Build history of the part. All positions in model axes, mm. A direction names the side the tool comes from. Round coordinates to 2 decimals unless told otherwise and drop trailing zeros. Loops run counter-clockwise (first coordinate to the right, second up) from the corner with the lowest first, then second, coordinate; pieces in that order, holes last. Notation, with made-up numbers: (-34.5, 50) -> (-1.5, 50) arc R20 cw to (-1.5, 80) -> close; hole circle Ø9 at (-22.5, 9). An arc over 180 degrees is marked (long way). Put each result on its own line as item: value. Start each with the question number.
Item 1: Cut at C-C, the plane y = 5. List the corners of the cut face in (x, z), plus the area to 3 significant figures.
Item 2: Flat gauge pins, fed straight in: pin 1 Ø5 at (y, z) = (15, -8.5) entering from -X; pin 2 Ø8.5 at (y, z) = (13.5, 8) entering from +X; pin 3 Ø1.9 at (x, z) = (41.5, -40.5) entering from +Y; pin 4 Ø5 at (x, z) = (25, 30.5) entering from -Y. Where does each tip first touch, or does it go through?
Item 3: Tool access for faces 5 (the flat face through (-1, 19, 38)), 6 (the flat face through (-36, 6, 32)), 7 (the flat face through (-39, 19, 1)): list every direction of +Z, -Z, +X, -X, +Y, -Y with a clear straight run to the whole face (end or side of a thin tool).
Item 4: Drill centre lines: probe 1 along Z at (x, y) = (25, 18.7); probe 2 along X at (y, z) = (17.7, 30.5); probe 3 along X at (y, z) = (0.95, -40.5). Where is each one in solid material? Low to high. Write a range as [from, to].
Item 5: Cut at B-B, the plane z = 30.5. List the corners of the cut face in (x, y).
Item 6: Cut at D-D, the plane x = 25. List the corners of the cut face in (y, z), plus the area to 3 significant figures.
Item 7: Cut at A-A, the plane x = 41.5. List the corners of the cut face in (y, z).
Item 8: Pull direction Z, two halves, no side cores. Call faces 1 (the cylindrical face through (-40.76, 1.52, -39.08)), 2 (the flat face through (39, 0, -38)), 3 (the flat face through (39, 1, -44)), 4 (the flat face through (-39, 1, 44)): +Z half, -Z half, draft (parallel to the pull), parting line (faces both ways), or undercut.
```python
from build123d import *

# Parameters (mm, degrees)
SKETCH1_W             = 12
SKETCH1_H             = 12
BOSS_EXTRUDE1_DEPTH   = 3
BOSS_EXTRUDE1_2_DEPTH = 3
BOSS_EXTRUDE1_3_DEPTH = 3
BOSS_EXTRUDE1_4_DEPTH = 3
SKETCH2_W             = 6
SKETCH2_H             = 6
BOSS_EXTRUDE3_DEPTH   = 14
SKETCH3_W             = 78
SKETCH3_H             = 76
BOSS_EXTRUDE4_DEPTH   = 3
CUT_EXTRUDE1_REACH    = 5
SKETCH4_R             = 1.6
CUT_EXTRUDE2_REACH    = 22
SKETCH5_R             = 2.1


with BuildPart() as part:
    # Sketch1 → Boss-Extrude1 (new body)
    with BuildSketch(Plane(origin=(0, 0, 0), x_dir=(1, 0, 0), z_dir=(0, 1, 0))):
        with Locations((-39, -38)):
            Rectangle(SKETCH1_W, SKETCH1_H)
    extrude(amount=BOSS_EXTRUDE1_DEPTH)



with BuildPart() as body_2:
    # Sketch1 → Boss-Extrude1 2 (new body)
    with BuildSketch(Plane(origin=(0, 0, 0), x_dir=(1, 0, 0), z_dir=(0, 1, 0))):
        with Locations((-39, 38)):
            Rectangle(SKETCH1_W, SKETCH1_H)
    extrude(amount=BOSS_EXTRUDE1_2_DEPTH)


with BuildPart() as body_3:
    # Sketch1 → Boss-Extrude1 3 (new body)
    with BuildSketch(Plane(origin=(0, 0, 0), x_dir=(1, 0, 0), z_dir=(0, 1, 0))):
        with Locations((39, 38)):
            Rectangle(SKETCH1_W, SKETCH1_H)
    extrude(amount=BOSS_EXTRUDE1_3_DEPTH)


with BuildPart() as body_4:
    # Sketch1 → Boss-Extrude1 4 (new body)
    with BuildSketch(Plane(origin=(0, 0, 0), x_dir=(1, 0, 0), z_dir=(0, 1, 0))):
        with Locations((39, -38)):
            Rectangle(SKETCH1_W, SKETCH1_H)
    extrude(amount=BOSS_EXTRUDE1_4_DEPTH)


with BuildPart() as part_1:
    add(part.part)

    add(body_2.part)  # Boss-Extrude3 merges body 2

    add(body_3.part)  # Boss-Extrude3 merges body 3

    add(body_4.part)  # Boss-Extrude3 merges body 4
    # Sketch2 → Boss-Extrude3 (add)
    with BuildSketch(Plane(origin=(0, 3, 0), x_dir=(1, 0, 0), z_dir=(0, 1, 0))):
        with Locations((-36, 35)):
            Rectangle(SKETCH2_W, SKETCH2_H)
        with Locations((-36, -35)):
            Rectangle(SKETCH2_W, SKETCH2_H)
        with Locations((36, 35)):
            Rectangle(SKETCH2_W, SKETCH2_H)
        with Locations((36, -35)):
            Rectangle(SKETCH2_W, SKETCH2_H)
    extrude(amount=BOSS_EXTRUDE3_DEPTH)

    # Sketch3 → Boss-Extrude4 (add)
    with BuildSketch(Plane(origin=(0, 17, 0), x_dir=(1, 0, 0), z_dir=(0, 1, 0))):
        Rectangle(SKETCH3_W, SKETCH3_H)
    extrude(amount=BOSS_EXTRUDE4_DEPTH)

    # Sketch4 → Cut-Extrude1 (cut, up to next)
    with BuildSketch(Plane(origin=(0, 3, 0), x_dir=(1, 0, 0), z_dir=(0, 1, 0)), mode=Mode.PRIVATE) as cut_extrude1_sk1:
        with Locations((41.5, -40.5)):
            Circle(SKETCH4_R)
    cut_extrude1_tool1 = extrude(cut_extrude1_sk1.sketch, amount=-CUT_EXTRUDE1_REACH, mode=Mode.PRIVATE) & part_1.part
    add(cut_extrude1_tool1.solids().sort_by_distance((41.5, 3, 40.5))[0], mode=Mode.SUBTRACT)
    # Sketch4 → Cut-Extrude1 (cut, up to next)
    with BuildSketch(Plane(origin=(0, 3, 0), x_dir=(1, 0, 0), z_dir=(0, 1, 0)), mode=Mode.PRIVATE) as cut_extrude1_sk2:
        with Locations((-41.5, 40.5)):
            Circle(SKETCH4_R)
    cut_extrude1_tool2 = extrude(cut_extrude1_sk2.sketch, amount=-CUT_EXTRUDE1_REACH, mode=Mode.PRIVATE) & part_1.part
    add(cut_extrude1_tool2.solids().sort_by_distance((-41.5, 3, -40.5))[0], mode=Mode.SUBTRACT)
    # Sketch4 → Cut-Extrude1 (cut, up to next)
    with BuildSketch(Plane(origin=(0, 3, 0), x_dir=(1, 0, 0), z_dir=(0, 1, 0)), mode=Mode.PRIVATE) as cut_extrude1_sk3:
        with Locations((-41.5, -40.5)):
            Circle(SKETCH4_R)
    cut_extrude1_tool3 = extrude(cut_extrude1_sk3.sketch, amount=-CUT_EXTRUDE1_REACH, mode=Mode.PRIVATE) & part_1.part
    add(cut_extrude1_tool3.solids().sort_by_distance((-41.5, 3, 40.5))[0], mode=Mode.SUBTRACT)
    # Sketch4 → Cut-Extrude1 (cut, up to next)
    with BuildSketch(Plane(origin=(0, 3, 0), x_dir=(1, 0, 0), z_dir=(0, 1, 0)), mode=Mode.PRIVATE) as cut_extrude1_sk4:
        with Locations((41.5, 40.5)):
            Circle(SKETCH4_R)
    cut_extrude1_tool4 = extrude(cut_extrude1_sk4.sketch, amount=-CUT_EXTRUDE1_REACH, mode=Mode.PRIVATE) & part_1.part
    add(cut_extrude1_tool4.solids().sort_by_distance((41.5, 3, -40.5))[0], mode=Mode.SUBTRACT)

    # Sketch5 → Cut-Extrude2 (cut, up to next)
    with BuildSketch(Plane(origin=(0, 20, 0), x_dir=(1, 0, 0), z_dir=(0, 1, 0)), mode=Mode.PRIVATE) as cut_extrude2_sk1:
        with Locations((25, 30.5)):
            Circle(SKETCH5_R)
    cut_extrude2_tool1 = extrude(cut_extrude2_sk1.sketch, amount=-CUT_EXTRUDE2_REACH, mode=Mode.PRIVATE) & part_1.part
    add(cut_extrude2_tool1.solids().sort_by_distance((25, 20, -30.5))[0], mode=Mode.SUBTRACT)
    # Sketch5 → Cut-Extrude2 (cut, up to next)
    with BuildSketch(Plane(origin=(0, 20, 0), x_dir=(1, 0, 0), z_dir=(0, 1, 0)), mode=Mode.PRIVATE) as cut_extrude2_sk2:
        with Locations((25, -30.5)):
            Circle(SKETCH5_R)
    cut_extrude2_tool2 = extrude(cut_extrude2_sk2.sketch, amount=-CUT_EXTRUDE2_REACH, mode=Mode.PRIVATE) & part_1.part
    add(cut_extrude2_tool2.solids().sort_by_distance((25, 20, 30.5))[0], mode=Mode.SUBTRACT)
    # Sketch5 → Cut-Extrude2 (cut, up to next)
    with BuildSketch(Plane(origin=(0, 20, 0), x_dir=(1, 0, 0), z_dir=(0, 1, 0)), mode=Mode.PRIVATE) as cut_extrude2_sk3:
        with Locations((-25, 30.5)):
            Circle(SKETCH5_R)
    cut_extrude2_tool3 = extrude(cut_extrude2_sk3.sketch, amount=-CUT_EXTRUDE2_REACH, mode=Mode.PRIVATE) & part_1.part
    add(cut_extrude2_tool3.solids().sort_by_distance((-25, 20, -30.5))[0], mode=Mode.SUBTRACT)
    # Sketch5 → Cut-Extrude2 (cut, up to next)
    with BuildSketch(Plane(origin=(0, 20, 0), x_dir=(1, 0, 0), z_dir=(0, 1, 0)), mode=Mode.PRIVATE) as cut_extrude2_sk4:
        with Locations((-25, -30.5)):
            Circle(SKETCH5_R)
    cut_extrude2_tool4 = extrude(cut_extrude2_sk4.sketch, amount=-CUT_EXTRUDE2_REACH, mode=Mode.PRIVATE) & part_1.part
    add(cut_extrude2_tool4.solids().sort_by_distance((-25, 20, 30.5))[0], mode=Mode.SUBTRACT)


solid = part_1.part
```
Reply:
1. outline: (-39, -38) -> (-33, -38) -> (-33, -32) -> (-39, -32) -> close; (-39, 32) -> (-33, 32) -> (-33, 38) -> (-39, 38) -> close; (33, -38) -> (39, -38) -> (39, -32) -> (33, -32) -> close; (33, 32) -> (39, 32) -> (39, 38) -> (33, 38) -> close
1. area: 144 mm^2
2. pin 1: stops at x = -39
2. pin 2: stops at x = 39
2. pin 3: passes through
2. pin 4: stops at y = 17
3. face 5: +Z, +X, -X, +Y
3. face 6: +X, -X, -Y
3. face 7: +Z, -Z, -X, +Y
4. probe 1: z = [-38, -32.6], [-28.4, 28.4], [32.6, 38]
4. probe 2: x = [-39, -27.1], [-22.9, 22.9], [27.1, 39]
4. probe 3: x = [-45, -43.1], [-39.9, -33], [33, 39.9], [43.1, 45]
5. outline: (-39, 17) -> (-27.1, 17) -> (-27.1, 20) -> (-39, 20) -> close; (-22.9, 17) -> (22.9, 17) -> (22.9, 20) -> (-22.9, 20) -> close; (27.1, 17) -> (39, 17) -> (39, 20) -> (27.1, 20) -> close
6. outline: (17, -38) -> (20, -38) -> (20, -32.6) -> (17, -32.6) -> close; (17, -28.4) -> (20, -28.4) -> (20, 28.4) -> (17, 28.4) -> close; (17, 32.6) -> (20, 32.6) -> (20, 38) -> (17, 38) -> close
6. area: 203 mm^2
7. outline: (0, -44) -> (3, -44) -> (3, -42.1) -> (0, -42.1) -> close; (0, -38.9) -> (3, -38.9) -> (3, -32) -> (0, -32) -> close; (0, 32) -> (3, 32) -> (3, 38.9) -> (0, 38.9) -> close; (0, 42.1) -> (3, 42.1) -> (3, 44) -> (0, 44) -> close
8. face 1: undercut
8. face 2: draft
8. face 3: -Z half
8. face 4: +Z half
